Read the model definition and answer for the solid it produces. Units are mm, in the model's axes. A direction names the side the tool comes from. Give positions to 0.01 mm unless a question says otherwise; leave off trailing zeros. Order: outer loops, then holes, each group sorted by start corner. A loop starts at its lowest first (then second) coordinate and runs counter-clockwise, first axis right, second up. Notation, with made-up numbers: (76.5, 29.5) - (105.5, 29.5) arc R22 cw to (105.5, 65.5) - close; hole circle Ø5 at (-28, 47). An arc over 180 degrees is marked (long way). Write each question's results on one line, items separated by ' | '. Start each with the question number.
Q1. A flat-ended cylindrical pin translates along its axis: P1, Ø8, axis at x = 24.5, z = -10.5, coming from the -Y side. Find the tip coordinate at first contact, or state that the pin passes through.
Q2. For a pull along Y with two mould halves and no side action, classify faces 1 (the face through (0, 2, -31)), 2 (the face through (45.001, -14.519, -54.008)), 3 (the face through (23, 4.978, -32)), 4 (the face through (45.13, -22.04, -23.107)) as +Y half, -Y half, draft (parallel to the pull), parting line (faces both ways), or undercut.
Q3. Find the intervals of material crossed by line 1 along Y through (x, z) = (35.5, -18); line 2 along X through (y, z) = (-1.5, -29.5), in increasing order. Write a range as from..to.
Q4. Find section C-C on y = -29. Give the vertices of the cut face in (x, z), and give its area (3 significant figures).
Q5. Find section A-A on x = 25.5. Give the vertices of the cut face in (y, z), and give its area (3 significant figures).
Q6. Find section B-B on z = -59. Give the vertices of the cut face in (x, y), and give its area (3 significant figures).
Q7. Find section D-D on z = -7. Give the vertices of the cut face in (x, y), and give its area (3 significant figures).
Q8. A tool of negligible diameter and unlimited length cuts with its end or side. For faces 5 (the face through (42.647, -5, -32)), 6 (the face through (47.422, -6, -32)), from which of +Z, -Z, +X, -X, +Y, -Y can it reach the whole face along a straight path? Write none if from no direction.
from build123d import *

# Parameters (mm, degrees)
SKETCH1_W           = 47.4218
SKETCH1_H           = 63.5762
BOSS_EXTRUDE1_DEPTH = 4.9784
SKETCH3_W           = 4.7752
SKETCH3_H           = 63.5762
BOSS_EXTRUDE2_DEPTH = 34.4424
SKETCH4_R           = 9.398
CUT_EXTRUDE1_DEPTH  = 5.7752
FILLET1_R           = 1.27
FILLET2_R           = 1.27
FILLET3_R           = 0.254


with BuildPart() as part:
    # Sketch1 → Boss-Extrude1 (new body)
    with BuildSketch(Plane(origin=(0, 0, 0), x_dir=(1, 0, 0), z_dir=(0, 1, 0))):
        with Locations((23.7109, 31.7881)):
            Rectangle(SKETCH1_W, SKETCH1_H)
    extrude(amount=BOSS_EXTRUDE1_DEPTH)

    # Sketch3 → Boss-Extrude2 (add)
    with BuildSketch(Plane.XZ):
        with Locations((45.0342, -31.7881)):
            Rectangle(SKETCH3_W, SKETCH3_H)
    extrude(amount=BOSS_EXTRUDE2_DEPTH)

    # Sketch4 → Cut-Extrude1 (cut, through all)
    with BuildSketch(Plane.ZY.offset(-42.6466)):
        with BuildLine():
            Line((0, -34.4424), (0, -0.762))
            Line((0, -0.762), (-18.65127846, -27.577572639))
            ThreePointArc((-18.65127846, -27.577572639), (-24.376927103, -32.622731271), (-31.7881, -34.4424))
            Line((-31.7881, -34.4424), (0, -34.4424))
        make_face()
        with BuildLine():
            Line((-44.92492154, -27.577572639), (-63.5762, -0.762))
            Line((-63.5762, -0.762), (-63.5762, -34.4424))
            Line((-63.5762, -34.4424), (-31.7881, -34.4424))
            ThreePointArc((-31.7881, -34.4424), (-39.199272897, -32.622731271), (-44.92492154, -27.577572639))
        make_face()
        with Locations((-31.7881, -18.4404)):
            Circle(SKETCH4_R)
    extrude(amount=-CUT_EXTRUDE1_DEPTH, mode=Mode.SUBTRACT)

    # Fillet1
    fillet1_edges = [part.edges().sort_by_distance(p)[0] for p in [
        (45.0342, -0.762, 0),
        (45.0342, -0.762, -63.5762),
    ]]
    fillet(fillet1_edges, radius=FILLET1_R)

    # Fillet2
    fillet2_edges = [part.edges().sort_by_distance(p)[0] for p in [
        (0, 2.4892, -63.5762),
        (0, 2.4892, 0),
    ]]
    fillet(fillet2_edges, radius=FILLET2_R)

    # Fillet3
    fillet3_edges = [part.edges().sort_by_distance(p)[0] for p in [
        (42.6466, -18.4404, -41.1861),
    ]]
    fillet(fillet3_edges, radius=FILLET3_R)


solid = part.part
Working result:
1) P1: y = 0
2) face 1: draft | face 2: -Y half | face 3: +Y half | face 4: undercut
3) line 1: 0..4.98 | line 2: 42.65..47.42
4) outline: (42.65, -43.81) - (47.42, -43.81) - (47.42, -19.76) - (42.65, -19.76) - close | area: 115 mm²
5) outline: (0, -63.58) - (4.98, -63.58) - (4.98, 0) - (0, 0) - close | area: 317 mm²
6) outline: (0, 0) - (42.65, 0) - (42.65, -7.34) - (47.42, -7.34) - (47.42, 4.98) - (0, 4.98) - close | area: 271 mm²
7) outline: (0, 0) - (42.65, 0) - (42.65, -10.83) - (47.42, -10.83) - (47.42, 4.98) - (0, 4.98) - close | area: 288 mm²
8) face 5: +Z, -Z, -X, -Y | face 6: +Z, -Z, +X, +Y, -Y
